from build123d import *

# Parameters (mm, degrees)
SKETCH_1_R      = 16
SKETCH_1_R_2    = 1.1
SKETCH_1_R_3    = 5.5
EXTRUDE_1_DEPTH = 3
SKETCH_2_R      = 14
SKETCH_2_R_2    = 13
EXTRUDE_2_DEPTH = 3
THREAD_1_PITCH  = 2
THREAD_1_FROM   = 2
CHAMFER_1_SIZE  = 1
CHAMFER_2_SIZE  = 1


with BuildPart() as part:
    # Sketch 1 → Бобышка-Вытянуть1 (new body)
    with BuildSketch(Plane(origin=(0, 0, 0), x_dir=(1, 0, 0), z_dir=(0, 1, 0))):
        with Locations(Location((0, 0, 0), (0, 0, 270))):
            Circle(SKETCH_1_R)
        with Locations(Location((0, 8.5, 0), (0, 0, 270))):
            Circle(SKETCH_1_R_2, mode=Mode.SUBTRACT)
        with Locations(Location((7.361215932, -4.25, 0), (0, 0, 270))):
            Circle(SKETCH_1_R_2, mode=Mode.SUBTRACT)
        with Locations(Location((-7.361215932, -4.25, 0), (0, 0, 270))):
            Circle(SKETCH_1_R_2, mode=Mode.SUBTRACT)
        with Locations(Location((0, 0, 0), (0, 0, 270))):
            Circle(SKETCH_1_R_3, mode=Mode.SUBTRACT)
    extrude(amount=EXTRUDE_1_DEPTH)

    # Эскиз2 → Бобышка-Вытянуть2 (add)
    with BuildSketch(Plane.XZ):
        with Locations(Location((0, 0, 0), (0, 0, 90))):
            Circle(SKETCH_2_R)
        with Locations(Location((0, 0, 0), (0, 0, 270))):
            Circle(SKETCH_2_R_2, mode=Mode.SUBTRACT)
    extrude(amount=EXTRUDE_2_DEPTH)

    # Резьба1: arcs per turn and ends read off the stored shape
    # Резьба1: the profile of Sketch 1 2 profile screwed along a right-hand helix through 2.5 turns, 10 arcs to a turn; built about Z, then put on its axis
    thread_1_z = Axis((0, 0, 0), (0, 0, 1))
    thread_1_corners = [(13.9997, 0, -0.000173205), (15.08253175, 0, 0.624999997), (15.08253175, 0, 0.874999997), (13.9997, 0, 1.5001732)]
    with BuildLine(mode=Mode.PRIVATE) as thread_1_profile:
        Line(thread_1_corners[0], thread_1_corners[1])
        Line(thread_1_corners[1], thread_1_corners[2])
        Line(thread_1_corners[2], thread_1_corners[3])
        Line(thread_1_corners[3], thread_1_corners[0])
    thread_1_cap = Face(thread_1_profile.wire())
    thread_1_turn_angles = [0, 18, 36, 54, 72, 90, 108, 126, 144, 162, 180, 198, 216, 234, 252, 270, 288, 306, 324, 342, 360]
    thread_1_turn_weights = [1, 0.9510565162951535, 1, 0.9510565162951535, 1, 0.9510565162951535, 1, 0.9510565162951535, 1, 0.9510565162951535, 1, 0.9510565162951535, 1, 0.9510565162951535, 1, 0.9510565162951535, 1, 0.9510565162951535, 1, 0.9510565162951535, 1]
    thread_1_turn_rails = [Edge.make_bspline([Vector(p[0], p[1], 0).rotate(thread_1_z, thread_1_turn_angles[k]) / thread_1_turn_weights[k] + Vector(0, 0, p[2] + THREAD_1_PITCH * thread_1_turn_angles[k] / 360) for k in range(21)], [0, 0, 0, 1, 1, 2, 2, 3, 3, 4, 4, 5, 5, 6, 6, 7, 7, 8, 8, 9, 9, 10, 10, 10], 2, thread_1_turn_weights) for p in thread_1_corners]
    thread_1_turn_sides = [Face.make_surface_from_curves(thread_1_turn_rails[p[0]], thread_1_turn_rails[p[1]]) for p in [(0, 1), (1, 2), (2, 3), (3, 0)]]
    thread_1_last_angles = [720, 738, 756, 774, 792, 810, 828, 846, 864, 882, 900]
    thread_1_last_weights = [1, 0.9510565162951535, 1, 0.9510565162951535, 1, 0.9510565162951535, 1, 0.9510565162951535, 1, 0.9510565162951535, 1]
    thread_1_last_rails = [Edge.make_bspline([Vector(p[0], p[1], 0).rotate(thread_1_z, thread_1_last_angles[k]) / thread_1_last_weights[k] + Vector(0, 0, p[2] + THREAD_1_PITCH * thread_1_last_angles[k] / 360) for k in range(11)], [0, 0, 0, 1, 1, 2, 2, 3, 3, 4, 4, 5, 5, 5], 2, thread_1_last_weights) for p in thread_1_corners]
    thread_1_last_sides = [Face.make_surface_from_curves(thread_1_last_rails[p[0]], thread_1_last_rails[p[1]]) for p in [(0, 1), (1, 2), (2, 3), (3, 0)]]
    thread_1 = Plane(origin=(0, -5, 0), x_dir=(1, 0, 0), z_dir=(0, 1, 0)) * split(Solid(Shell([*[p.moved(Location((0, 0, THREAD_1_PITCH * i))) for i in range(2) for p in thread_1_turn_sides], *thread_1_last_sides, thread_1_cap, thread_1_cap.rotate(thread_1_z, 900).moved(Location((0, 0, THREAD_1_PITCH * 900 / 360)))])), bisect_by=Plane.XY.offset(THREAD_1_FROM), keep=Keep.TOP, mode=Mode.PRIVATE)
    add(thread_1)

    # Фаска1
    chamfer_1_edges = [part.edges().sort_by_distance(p)[0] for p in [
        (7.361215932, 0, 3.15),
        (-7.361215932, 0, 3.15),
        (0, 3, -16),
        (0, 0, -9.6),
        (0, 3, -5.5),
    ]]
    chamfer(chamfer_1_edges, length=CHAMFER_1_SIZE)

    # Фаска2
    # the kernel refuses this chamfer: 1 mm, written as the material it takes off along each edge
    with BuildSketch(Plane(origin=(0, 0, 0), x_dir=(0, 0, 1), z_dir=(-1, 0, 0))) as chamfer_2_piece_1:
        Polygon((5.5, CHAMFER_2_SIZE), (5.5 + CHAMFER_2_SIZE, 0), (5.5, 0), align=None)
    revolve(axis=Axis((0, 0, 0), (0, 1, 0)), mode=Mode.SUBTRACT)


solid = part.part
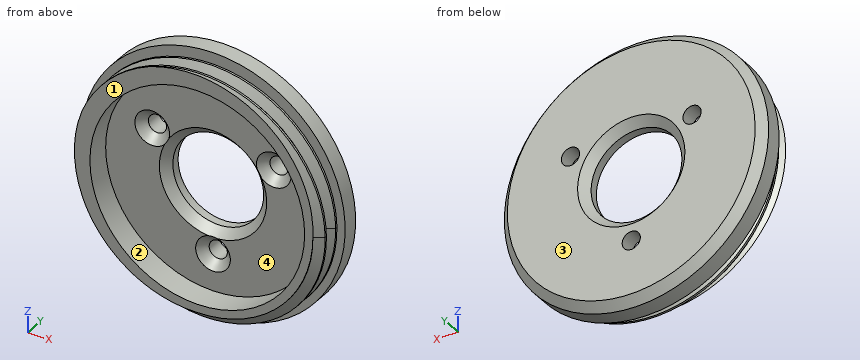
Design review of the part built by this model. Coordinates are the model's own, in mm. Face numbers are marked on the shaded views. A direction names the side the tool comes from. Give positions to 0.01 mm unless a question says otherwise; leave off trailing zeros. Order: outer loops, then holes, each group sorted by start corner. A loop starts at its lowest first (then second) coordinate and runs counter-clockwise, first axis right, second up. Notation, with made-up numbers: (46, 16.5) - (61, 16.5) arc R22 cw to (61, 53.5) - close; hole circle Ø9 at (0.25, 33). An arc over 180 degrees is marked (long way). Write item = value, one per line. Start each with the question number.
Q1. We need section A-A on y = 0.5. State the section outline as (x, z) points, plus the area to 3 significant figures.
Q2. Clearance check with flat-ended pins moving along their axes: pin 1 Ø13 at (x, z) = (4, -1) entering from -Y; pin 2 Ø1 at (y, z) = (0, 2) entering from -X; pin 3 Ø1.5 at (x, y) = (6, -1.5) entering from -Z. State where each tip first meets the part, or that it passes through.
Q3. Mouldability with a two-part tool opening along X and no side actions: class the marked faces 1 and 2 as released by +X, released by -X, zero draft, split by the parting line, or undercut.
Q4. Tool access review of the marked faces 3 and 4: name each direction out of +Z, -Z, +X, -X, +Y, -Y from which nothing blocks a thin tool from reaching the whole face with its end or side.
Q5. We need section B-B on z = 4.25. State how many separate pieces and enclosed holes the cut face has, plus the area to 3 significant figures.
Q6. To check wall thickness, follow L1, parallel to X at y = 1.4, z = 0; L2, parallel to X at y = 1.8, z = 4.25; L3, parallel to Y at x = 1, z = 14.5. State the ranges of each line that lie inside material, in increasing order. Write a range as from..to.
Working result:
q1.outline = circle Ø32 at (0, 0); hole circle Ø3.2 at (-7.36, 4.25); hole circle Ø12 at (0, 0); hole circle Ø3.2 at (0, -8.5); hole circle Ø3.2 at (7.36, 4.25)
q1.area = 667 mm²
q2.pin_1 = 0
q2.pin_2 = -15.93
q2.pin_3 = -14.12
q3.face_1 = zero draft
q3.face_2 = undercut
q4.face_3 = +Z, -Z, +X, -X, +Y
q4.face_4 = -Y
q5.separate_pieces = 4
q5.enclosed_holes = 0
q5.area = 61.9 mm²
q6.L1 = -16..-5.5, 5.5..16
q6.L2 = -15.43..-8.46, -6.26..-3.49, 3.49..6.26, 8.46..15.43
q6.L3 = -3..-2.29, -1.17..-0.29, 0..3
